```python
from build123d import *

# Parameters (mm, degrees)
SKETCH1_R           = 3.4925
SKETCH1_R_2         = 3.175
BOSS_EXTRUDE1_DEPTH = 3.175
FILLET2_R           = 2.54
FILLET3_R           = 2.54
SKETCH4_W           = 25.4
SKETCH4_H           = 7.62
CUT_EXTRUDE1_DEPTH  = 172.355687034
FILLET4_R           = 2.54


with BuildPart() as part:
    # Sketch1 → Boss-Extrude1 (new body)
    with BuildSketch(Plane.XY):
        Polygon((-57.15, -3.175), (-57.15, 15.875), (57.15, 15.875), (57.15, -1.009681966), (73.025, -1.009681966), (73.025, -27.559), (73.025, -154.983999912), (-73.025, -154.983999912), (-73.025, -27.559), (-73.025, -3.175), align=None)
        with Locations((-44.45, 6.35)):
            Circle(SKETCH1_R, mode=Mode.SUBTRACT)
        with Locations((44.45, 6.35)):
            Circle(SKETCH1_R, mode=Mode.SUBTRACT)
        with Locations((-63.5, -12.7)):
            Circle(SKETCH1_R_2, mode=Mode.SUBTRACT)
        with Locations((-38.1, -12.7)):
            Circle(SKETCH1_R_2, mode=Mode.SUBTRACT)
        with Locations((-12.7, -12.7)):
            Circle(SKETCH1_R_2, mode=Mode.SUBTRACT)
        with Locations((12.7, -12.7)):
            Circle(SKETCH1_R_2, mode=Mode.SUBTRACT)
        with Locations((38.1, -12.7)):
            Circle(SKETCH1_R_2, mode=Mode.SUBTRACT)
        with Locations((63.5, -12.7)):
            Circle(SKETCH1_R_2, mode=Mode.SUBTRACT)
        with Locations((-63.5, -105.199999912)):
            Circle(SKETCH1_R_2, mode=Mode.SUBTRACT)
        with Locations((-38.1, -105.199999912)):
            Circle(SKETCH1_R_2, mode=Mode.SUBTRACT)
        with Locations((-12.7, -105.199999912)):
            Circle(SKETCH1_R_2, mode=Mode.SUBTRACT)
        with Locations((12.7, -105.199999912)):
            Circle(SKETCH1_R_2, mode=Mode.SUBTRACT)
        with Locations((38.1, -105.199999912)):
            Circle(SKETCH1_R_2, mode=Mode.SUBTRACT)
        with Locations((63.5, -105.199999912)):
            Circle(SKETCH1_R_2, mode=Mode.SUBTRACT)
    extrude(amount=BOSS_EXTRUDE1_DEPTH)

    # Fillet2
    fillet2_edges = [part.edges().sort_by_distance(p)[0] for p in [
        (-73.025, -154.983999912, 1.5875),
        (-73.025, -3.175, 1.5875),
        (-57.15, 15.875, 1.5875),
        (57.15, 15.875, 1.5875),
        (73.025, -1.009681966, 1.5875),
        (73.025, -154.983999912, 1.5875),
    ]]
    fillet(fillet2_edges, radius=FILLET2_R)

    # Fillet3
    fillet3_edges = [part.edges().sort_by_distance(p)[0] for p in [
        (-57.15, -3.175, 1.5875),
        (57.15, -1.009681966, 1.5875),
    ]]
    fillet(fillet3_edges, radius=FILLET3_R)

    # Sketch4 → Cut-Extrude1 (cut, through all)
    with BuildSketch(Plane(origin=(0, 0, 0), x_dir=(-1, 0, 0), z_dir=(0, 0, -1))):
        with Locations((-12.7, -148.633999912)):
            Rectangle(SKETCH4_W, SKETCH4_H)
    extrude(amount=-CUT_EXTRUDE1_DEPTH, mode=Mode.SUBTRACT)

    # Fillet4
    fillet4_edges = [part.edges().sort_by_distance(p)[0] for p in [
        (0, -144.823999912, 1.5875),
        (0, -152.443999912, 1.5875),
        (25.4, -152.443999912, 1.5875),
        (25.4, -144.823999912, 1.5875),
    ]]
    fillet(fillet4_edges, radius=FILLET4_R)


solid = part.part
```
Build history of the part. All positions in model axes, mm. Give positions to 0.01 mm unless a question says otherwise; leave off trailing zeros. Loops run counter-clockwise (first coordinate to the right, second up) from the corner with the lowest first, then second, coordinate; pieces in that order, holes last. Notation, with made-up numbers: (5, -6.5) -> (58, -6.5) arc R34 ccw to (58, 24.5) -> close; hole circle Ø6 at (53, 64). An arc over 180 degrees is marked (long way). One line per question, with ' | ' between items. Start each with the question number.
1) Cut at C-C (x = 12.7). Give the cut face in (y, z) (3 decimals), plus the area to 3 significant figures.
2) Two-plate mould, pull along X, no slides. Class faces 1 (the cylindrical face through (-41.27, -12.56, 1.57)), 2 (the flat face through (1, -68, 3.175)): released by +X, released by -X, zero draft, split by the parting line, or undercut.
3) Cut at B-B (y = -105.2). Give the cut face in (x, z) (3 decimals), plus the area to 3 significant figures.
4) Cut at D-D (y = 6.35). Count the separate pieces of the cut face and the enclosed holes in it, plus the area to 3 significant figures.
5) Cut at A-A (x = -12.7). Give the cut face in (y, z) (3 decimals), plus the area to 3 significant figures.
6) Pin check, flat tips, straight feed: pin 1 (4 mm diameter, centred on x = -12.7, y = -105.2, fed in from +Z); pin 2 (8 mm diameter, centred on x = -44.45, y = 6.35, fed in from +Z) (3 decimals); pin 3 (1 mm diameter, centred on y = 6, z = 1, fed in from +X); pin 4 (1.6 mm diameter, centred on x = -64.5, z = 1, fed in from +Y) (3 decimals). Stop position of each tip, or through.
7) Probe L1, parallel to Y at x = -12.7, z = 2.3 (3 decimals); L2, parallel to Y at x = -63.5, z = 2 (3 decimals); L3, parallel to Y at x = 12.7, z = 0.9 (3 decimals). List the from-to ranges inside material, lowest first.
Return value:
1) outline: (-154.984, 0) -> (-152.444, 0) -> (-152.444, 3.175) -> (-154.984, 3.175) -> close; (-144.824, 0) -> (-108.375, 0) -> (-108.375, 3.175) -> (-144.824, 3.175) -> close; (-102.025, 0) -> (-15.875, 0) -> (-15.875, 3.175) -> (-102.025, 3.175) -> close; (-9.525, 0) -> (15.875, 0) -> (15.875, 3.175) -> (-9.525, 3.175) -> close | area: 478 mm^2
2) face 1: undercut | face 2: zero draft
3) outline: (-73.025, 0) -> (-66.675, 0) -> (-66.675, 3.175) -> (-73.025, 3.175) -> close; (-60.325, 0) -> (-41.275, 0) -> (-41.275, 3.175) -> (-60.325, 3.175) -> close; (-34.925, 0) -> (-15.875, 0) -> (-15.875, 3.175) -> (-34.925, 3.175) -> close; (-9.525, 0) -> (9.525, 0) -> (9.525, 3.175) -> (-9.525, 3.175) -> close; (15.875, 0) -> (34.925, 0) -> (34.925, 3.175) -> (15.875, 3.175) -> close; (41.275, 0) -> (60.325, 0) -> (60.325, 3.175) -> (41.275, 3.175) -> close; (66.675, 0) -> (73.025, 0) -> (73.025, 3.175) -> (66.675, 3.175) -> close | area: 343 mm^2
4) separate pieces: 3 | enclosed holes: 0 | area: 319 mm^2
5) outline: (-154.984, 0) -> (-108.375, 0) -> (-108.375, 3.175) -> (-154.984, 3.175) -> close; (-102.025, 0) -> (-15.875, 0) -> (-15.875, 3.175) -> (-102.025, 3.175) -> close; (-9.525, 0) -> (15.875, 0) -> (15.875, 3.175) -> (-9.525, 3.175) -> close | area: 502 mm^2
6) pin 1: through | pin 2: z = 3.175 | pin 3: x = 57.15 | pin 4: y = -3.175
7) L1: -154.984 to -108.375, -102.025 to -15.875, -9.525 to 15.875 | L2: -154.984 to -108.375, -102.025 to -15.875, -9.525 to -3.175 | L3: -154.984 to -152.444, -144.824 to -108.375, -102.025 to -15.875, -9.525 to 15.875
